```python
from build123d import *

# Parameters (mm, degrees)
PAD010_DEPTH            = 200
FILLET035_R             = 5
FILLET034_R             = 5
FILLET036_R             = 5
SKETCH016_W             = 62.643768
SKETCH016_H             = 186.051987
POCKET_DEPTH            = 200
BODY006_ROLL_ANGLE      = 90
BODY006_PLACEMENT_ANGLE = 180


with BuildPart() as part:
    # Sketch017 → Pad010 (new body)
    with BuildSketch(Plane.XY):
        Polygon((0, 0), (145, 0), (145, 200), (68, 200), align=None)
    extrude(amount=PAD010_DEPTH)

    # Fillet035
    fillet035_edges = [part.edges().sort_by_distance(p)[0] for p in [
        (34, 100, 0),
        (34, 100, 200),
    ]]
    fillet(fillet035_edges, radius=FILLET035_R)

    # Fillet034
    fillet034_edges = [part.edges().sort_by_distance(p)[0] for p in [
        (145, 100, 0),
    ]]
    fillet(fillet034_edges, radius=FILLET034_R)

    # Fillet036
    fillet036_edges = [part.edges().sort_by_distance(p)[0] for p in [
        (145, 100, 200),
    ]]
    fillet(fillet036_edges, radius=FILLET036_R)

    # Sketch016 (on Face10 of Fillet036) → Pocket (cut)
    with BuildSketch(Plane(origin=(0, 200, 0), x_dir=(-1, 0, 0), z_dir=(0, 1, 0))):
        with Locations((-106.638336, 100.319633)):
            Rectangle(SKETCH016_W, SKETCH016_H)
    extrude(amount=-POCKET_DEPTH, mode=Mode.SUBTRACT)


with BuildPart() as part_1:
    # Body006 roll: moved
    add(part.part.rotate(Axis((0, 0, 0), (1, 0, 0)), BODY006_ROLL_ANGLE))


with BuildPart() as part_2:
    # Body006 placement: moved
    add(part_1.part.moved(Location((-170, -92, -9))).rotate(Axis((-170, -92, -9), (0, 0, 1)), BODY006_PLACEMENT_ANGLE))


solid = part_2.part
```
Can you work these out from the model? Positions are in its coordinate system, mm. A direction names the side the tool comes from. Give positions to 0.01 mm unless a question says otherwise; leave off trailing zeros. Write each loop counter-clockwise with the first axis right and the second up, starting at its lowest first coordinate (ties: lowest second). Pieces come first, ordered by that corner, then holes. Notation, with made-up numbers: (-14, 74) -> (-1, 74) arc R8 ccw to (-1, 80) -> close; hole circle Ø2 at (54.25, 41.5). An arc over 180 degrees is marked (long way). One line per item, written item: value.
Q1. Please list where these lines run through material, in increasing order: line 1 (Y direction, x = -286, z = 82.5); line 2 (X direction, y = 82.5, z = 163); line 3 (X direction, y = 49, z = 118). Write a range as [from, to].
Results found:
line 1: y = [-92, -84.71], [101.35, 108]
line 2: x = [-315, -307.96], [-245.32, -228.48]
line 3: x = [-315, -307.96], [-245.32, -213.18]
Q2. Imagine slicing it at B-B on y = -1. Please give me the cut outline in (x, z).
Results found:
outline: (-315, -9) -> (-307.96, -9) -> (-307.96, 191) -> (-315, 191) -> close; (-245.32, -9) -> (-170, -9) -> (-238, 191) -> (-245.32, 191) -> close
Q3. Which directions (+Z, -Z, +X, -X, +Y, -Y) give clear straight access to the entire face, cutting with the end or side of a thin tool? Please do faces 1 (the face through (-277, 101.346, 92)), 2 (the face through (-257, -92, 92)).
Results found:
face 1: +Z, -Z
face 2: +Z, -Z, +X, -X, -Y
Q4. Imagine slicing it at A-A on x = -252.5. Please give me the cut outline in (y, z).
Results found:
outline: (-92, -9) -> (-84.71, -9) -> (-84.71, 191) -> (-92, 191) -> close; (101.35, -9) -> (108, -9) -> (108, 191) -> (101.35, 191) -> close
Q5. We'd pull the mould along Y, two halves only. Please class faces 3 (the face through (-204.476, 6.67, 92.4)), 4 (the face through (-277, -84.706, 92)), 5 (the face through (-313, -91, 92)), 6 (the face through (-245.316, 7, 92)): +Y half, -Y half, draft (parallel to the pull), parting line (faces both ways), or undercut.
Results found:
face 3: draft
face 4: undercut
face 5: -Y half
face 6: undercut
